The listing builds one solid part. Answer for the finished solid, in the listing's coordinates (mm). Face numbers are marked on the shaded views. A direction names the side the tool comes from. Coordinates: 2 decimals unless noted, no trailing zeros. Loops run counter-clockwise (first coordinate to the right, second up) from the corner with the lowest first, then second, coordinate; pieces in that order, holes last. Notation, with made-up numbers: (38, 21) -> (58, 21) arc R14 ccw to (58, 33) -> close; hole circle Ø7 at (69.5, 5.25). An arc over 180 degrees is marked (long way). Answer in a Markdown table with one row per item.
```python
from build123d import *

# Parameters (mm, degrees)
BASPROSKE_W        = 12
BASPROSKE_H        = 55.25
TOOTHCUT_DEPTH     = 80.051407325
TEETHCUTS_COUNT    = 15
TEETHCUTS_ANGLE    = 336
BORSKE_R           = 10
BORE_DEPTH         = 50.0000508
SKETCH1_W          = 31
SKETCH1_H          = 31
CUT_EXTRUDE2_DEPTH = 79.934396957
FILLET1_R          = 2


with BuildPart() as part:
    # BasProSke → Base-Revolve (revolve)
    with BuildSketch(Plane(origin=(0, 0, 0), x_dir=(1, 0, 0), z_dir=(0, 1, 0)), mode=Mode.PRIVATE) as base_revolve_sk:
        with Locations((6, 27.625)):
            Rectangle(BASPROSKE_W, BASPROSKE_H)
    revolve(base_revolve_sk.sketch.rotate(Axis((-10, 0, 0), (1, 0, 0)), 180), axis=Axis((-10, 0, 0), (1, 0, 0)))

    # TooCutSke → ToothCut (cut, through all)
    with BuildSketch(Plane(origin=(0, 0, 0), x_dir=(0, 0, -1), z_dir=(1, 0, 0))):
        with BuildLine():
            ThreePointArc((3.414601006, 40.480240562), (0, 40.624), (-3.414601006, 40.480240562))
            ThreePointArc((-3.414601006, 40.480240562), (-5.310758866, 48.09911095), (-10.058002941, 54.352611915))
            ThreePointArc((-10.058002941, 54.352611915), (0, 55.2754), (10.058002941, 54.352611915))
            ThreePointArc((10.058002941, 54.352611915), (5.310758866, 48.09911095), (3.414601006, 40.480240562))
        make_face()
    toothcut = extrude(amount=TOOTHCUT_DEPTH, mode=Mode.SUBTRACT)

    # TeethCuts: ToothCut ×15 about axis
    teethcuts_axis = Axis((-10, 0, 0), (1, 0, 0))
    for i in range(1, TEETHCUTS_COUNT):
        add(toothcut.rotate(teethcuts_axis, i * TEETHCUTS_ANGLE / (TEETHCUTS_COUNT - 1)), mode=Mode.SUBTRACT)

    # BorSke → Bore (cut, symmetric)
    with BuildSketch(Plane(origin=(0, 0, 0), x_dir=(0, 0, -1), z_dir=(1, 0, 0))):
        with Locations(Location((0, 0, 0), (0, 0, 180))):
            Circle(BORSKE_R)
    extrude(amount=BORE_DEPTH, both=True, mode=Mode.SUBTRACT)

    # Sketch1 → Cut-Extrude2 (cut, through all)
    with BuildSketch(Plane(origin=(12, 0, 0), x_dir=(0, 0, -1), z_dir=(1, 0, 0))):
        Rectangle(SKETCH1_W, SKETCH1_H)
    extrude(amount=-CUT_EXTRUDE2_DEPTH, mode=Mode.SUBTRACT)

    # Fillet1
    fillet1_edges = [part.edges().sort_by_distance(p)[0] for p in [
        (0, 0, -15.5),
        (6, 15.5, -15.5),
        (0, -15.5, 0),
        (6, -15.5, -15.5),
        (0, 0, 15.5),
        (6, -15.5, 15.5),
        (0, 15.5, 0),
        (6, 15.5, 15.5),
        (12, 0, -15.5),
        (12, 15.5, 0),
        (12, 0, 15.5),
        (12, -15.5, 0),
    ]]
    fillet(fillet1_edges, radius=FILLET1_R)


solid = part.part
```
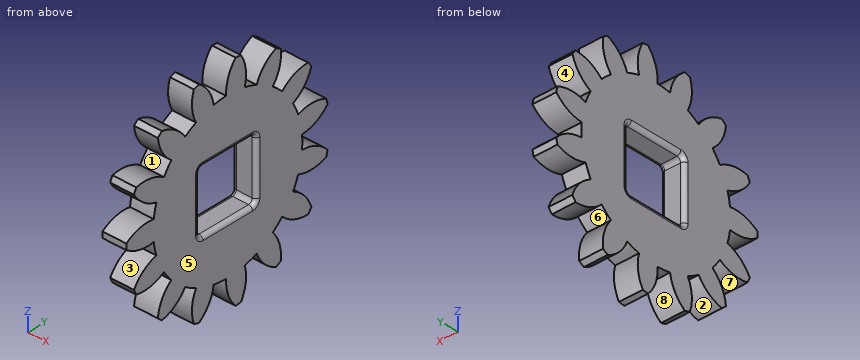
Item 1: Flat-ended cylindrical pins translate along their axes: pin 1 Ø4 at (x, y) = (4.5, 3.5) entering from +Z; pin 2 Ø3 at (x, z) = (6, -16.5) entering from -Y; pin 3 Ø5 at (x, y) = (5, 9) entering from -Z. Find the tip coordinate at first contact, or state that the pin passes through.
Findings below:
| item | result |
|---|---|
| pin 1 | stops at z = 55.08 |
| pin 2 | stops at y = -48.89 |
| pin 3 | stops at z = -54.87 |
Item 2: Determine the mould class of the marked faces 5, 6, 7 and 8 for opening direction Z: +Z half, -Z half, draft (parallel to the pull), parting line (faces both ways), or undercut.
Findings below:
| item | result |
|---|---|
| face 5 | draft |
| face 6 | undercut |
| face 7 | undercut |
| face 8 | -Z half |
Item 3: A cutting plane is placed at B-B, the plane z = -35. Determine the outline of the cut face in (x, y).
Findings below:
| item | result |
|---|---|
| outline | (0, -36.9) -> (12, -36.9) -> (12, -24.37) -> (0, -24.37) -> close; (0, -20.62) -> (12, -20.62) -> (12, 26.39) -> (0, 26.39) -> close |
Item 4: A tool of negligible diameter and unlimited length cuts with its end or side. For the marked faces 1, 2, 3 and 4, from which of +Z, -Z, +X, -X, +Y, -Y can it reach the whole face along a straight path? Write none if from no direction.
Findings below:
| item | result |
|---|---|
| face 1 | +X, -X |
| face 2 | -Z, +X, -X |
| face 3 | +X, -X, -Y |
| face 4 | +X, -X, +Y |
Item 5: Find the intervals of material crossed by probe 1 along Y at (x, z) = (1.25, 41); probe 2 along Z at (x, y) = (0.5, -50); probe 3 along Z at (x, y) = (11, -34.5), in increasing order.
Findings below:
| item | result |
|---|---|
| probe 1 | y = -37.03 to -32.38, -18.91 to -7.82, -0.86 to 9.61, 17.51 to 28.66 |
| probe 2 | z = -23.51 to -19.43, -4.26 to 4.26, 19.43 to 23.51 |
| probe 3 | z = -41.71 to -30.5, -21.45 to 21.45, 30.5 to 41.71 |
Item 6: A cutting plane is placed at A-A, the plane y = -6. Determine the outline of the cut face in (x, z).
Findings below:
| item | result |
|---|---|
| outline | (0, -40.18) -> (12, -40.18) -> (12, -17.5) arc R2 ccw to (10, -15.5) -> (2, -15.5) arc R2 ccw to (0, -17.5) -> close; (0, 17.5) arc R2 ccw to (2, 15.5) -> (10, 15.5) arc R2 ccw to (12, 17.5) -> (12, 40.18) -> (0, 40.18) -> close |
Item 7: A cutting plane is placed at C-C, the plane y = -27.5. Determine the outline of the cut face in (x, z), plus the area to 3 significant figures.
Findings below:
| item | result |
|---|---|
| outline | (0, -38.15) -> (12, -38.15) -> (12, 38.15) -> (0, 38.15) -> close |
| area | 916 mm2 |
